```python
from build123d import *

# Parameters (mm, degrees)
SKETCH001_W           = 9.26
SKETCH001_H           = 10.18
EXTRUDE001_DEPTH      = 1.355
EXTRUDE001_DEPTH_BACK = 0.3
SKETCH002_W           = 9.26
SKETCH002_H           = 10.18
EXTRUDE002_DEPTH      = 1.35
EXTRUDE002_DEPTH_BACK = 0.3
SKETCH003_R           = 0.3
EXTRUDE003_DEPTH      = 4
EXTRUDE_DEPTH         = 59.5


with BuildPart() as extrude001:
    # Sketch001 (on Face14 of Extrude) → Extrude001 (new body, two sides)
    with BuildSketch(Plane.XY.offset(59.5)) as extrude001_sk:
        with Locations((0, 10.39)):
            Rectangle(SKETCH001_W, SKETCH001_H)
    extrude(amount=EXTRUDE001_DEPTH)
    extrude(extrude001_sk.sketch, amount=-EXTRUDE001_DEPTH_BACK)


with BuildPart() as extrude002:
    # Sketch002 (on Face13 of Extrude) → Extrude002 (new body, two sides)
    with BuildSketch(Plane(origin=(0, 0, 0), x_dir=(1, 0, 0), z_dir=(0, 0, -1))) as extrude002_sk:
        with Locations((0, -10.39)):
            Rectangle(SKETCH002_W, SKETCH002_H)
    extrude(amount=EXTRUDE002_DEPTH)
    extrude(extrude002_sk.sketch, amount=-EXTRUDE002_DEPTH_BACK)


with BuildPart() as extrude003:
    # Sketch003 (on Face4 of Extrude) → Extrude003 (new body)
    with BuildSketch(Plane.XZ):
        with Locations((-2.54, 56.42)):
            Circle(SKETCH003_R)
        with Locations((-2.54, 53.88)):
            Circle(SKETCH003_R)
        with Locations((-2.54, 51.34)):
            Circle(SKETCH003_R)
        with Locations((-2.54, 48.8)):
            Circle(SKETCH003_R)
        with Locations((-2.54, 46.26)):
            Circle(SKETCH003_R)
        with Locations((-2.54, 43.72)):
            Circle(SKETCH003_R)
        with Locations((-2.54, 41.18)):
            Circle(SKETCH003_R)
        with Locations((-2.54, 38.64)):
            Circle(SKETCH003_R)
        with Locations((-2.54, 36.1)):
            Circle(SKETCH003_R)
        with Locations((-2.54, 33.56)):
            Circle(SKETCH003_R)
        with Locations((-2.54, 31.02)):
            Circle(SKETCH003_R)
        with Locations((-2.54, 28.48)):
            Circle(SKETCH003_R)
        with Locations((-2.54, 25.94)):
            Circle(SKETCH003_R)
        with Locations((-2.54, 23.4)):
            Circle(SKETCH003_R)
        with Locations((2.54, 23.4)):
            Circle(SKETCH003_R)
        with Locations((2.54, 25.94)):
            Circle(SKETCH003_R)
        with Locations((2.54, 28.48)):
            Circle(SKETCH003_R)
        with Locations((2.54, 31.02)):
            Circle(SKETCH003_R)
        with Locations((2.54, 33.56)):
            Circle(SKETCH003_R)
        with Locations((2.54, 36.1)):
            Circle(SKETCH003_R)
        with Locations((2.54, 38.64)):
            Circle(SKETCH003_R)
        with Locations((2.54, 41.18)):
            Circle(SKETCH003_R)
        with Locations((2.54, 43.72)):
            Circle(SKETCH003_R)
        with Locations((2.54, 46.26)):
            Circle(SKETCH003_R)
        with Locations((2.54, 48.8)):
            Circle(SKETCH003_R)
        with Locations((2.54, 51.34)):
            Circle(SKETCH003_R)
        with Locations((2.54, 53.88)):
            Circle(SKETCH003_R)
        with Locations((2.54, 56.42)):
            Circle(SKETCH003_R)
        with Locations((2.54, 10.7)):
            Circle(SKETCH003_R)
        with Locations((2.54, 13.24)):
            Circle(SKETCH003_R)
        with Locations((2.54, 15.78)):
            Circle(SKETCH003_R)
        with Locations((2.54, 18.32)):
            Circle(SKETCH003_R)
        with Locations((2.54, 20.86)):
            Circle(SKETCH003_R)
        with Locations((2.54, 3.08)):
            Circle(SKETCH003_R)
        with Locations((2.54, 5.62)):
            Circle(SKETCH003_R)
        with Locations((2.54, 8.16)):
            Circle(SKETCH003_R)
        with Locations((-2.54, 10.7)):
            Circle(SKETCH003_R)
        with Locations((-2.54, 13.24)):
            Circle(SKETCH003_R)
        with Locations((-2.54, 15.78)):
            Circle(SKETCH003_R)
        with Locations((-2.54, 18.32)):
            Circle(SKETCH003_R)
        with Locations((-2.54, 20.86)):
            Circle(SKETCH003_R)
        with Locations((-2.54, 3.08)):
            Circle(SKETCH003_R)
        with Locations((-2.54, 5.62)):
            Circle(SKETCH003_R)
        with Locations((-2.54, 8.16)):
            Circle(SKETCH003_R)
    extrude(amount=EXTRUDE003_DEPTH)


with BuildPart() as fusion:
    # Sketch → Extrude (new body)
    with BuildSketch(Plane.XY):
        Polygon((-4.63, 15.48), (-4.63, 5.3), (-3.735, 5.3), (-3.735, 0), (3.735, 0), (3.735, 5.3), (4.63, 5.3), (4.63, 15.48), (1.17, 15.48), (1.17, 8.6), (-1.17, 8.6), (-1.17, 15.48), align=None)
    extrude(amount=EXTRUDE_DEPTH)

    # Fusion: union Extrude001, Extrude002, Extrude003
    add(extrude001.part)
    add(extrude002.part)
    add(extrude003.part)


solid = fusion.part
```
Source: CAD feature listing. Evaluate the final solid. Frame: model axes, mm. A direction names the side the tool comes from. Round coordinates to 2 decimals unless told otherwise and drop trailing zeros. Loops run counter-clockwise (first coordinate to the right, second up) from the corner with the lowest first, then second, coordinate; pieces in that order, holes last.
1. Section query C-C on z = 4. Output: boundary loops of the cut face in (x, y) (3 decimals), and give its area (3 significant figures).
2. Section query A-A on y = 10.5. Output: boundary loops of the cut face in (x, z) (3 decimals), and give its area (3 significant figures).
3. Mould query, pull axis X, two halves, no side actions, for faces 1 (the flat face through (0, 10, 60.855)), 2 (the flat face through (0, 12, 59.2)), 3 (the flat face through (-4.63, 10, 29)). Classes: released by +X, released by -X, zero draft, split by the parting line, or undercut.
4. Access query for faces 4 (the flat face through (0, 3, 0)), 5 (the flat face through (0, 12, 0.3)), 6 (the flat face through (0, 0, 29)), 7 (the flat face through (3.735, 3, 29)), 8 (the flat face through (0, 3, 59.5)). Directions: +Z, -Z, +X, -X, +Y, -Y. A direction counts if a zero-diameter tool reaches every point of the face in a straight line with its end or side. Return the directions, or none.
5. Section query D-D on y = -2.25. Give the number of separate pieces and of enclosed holes in the cut face, and give its area (3 significant figures).
6. Ray query, L1, parallel to X at y = 11.5, z = 41; L2, parallel to Y at x = 4, z = 36; L3, parallel to Y at x = 0.25, z = 17. Return the intervals inside material, ascending.
7. Section query B-B on x = -0.5. Output: boundary loops of the cut face in (y, z) (3 decimals).
8. Contact query for flat-ended pins moving along their axis: pin 1 (1.2 mm diameter, centred on x = 0, z = 40.5, fed in from +Y); pin 2 (4 mm diameter, centred on x = -0.5, y = 2.5, fed in from +Z); pin 3 (3 mm diameter, centred on y = -1, z = 30.5, fed in from -X) (3 decimals). Output: stop coordinate, or through.
Answers below:
1. outline: (-4.63, 5.3) - (-3.735, 5.3) - (-3.735, 0) - (3.735, 0) - (3.735, 5.3) - (4.63, 5.3) - (4.63, 15.48) - (1.17, 15.48) - (1.17, 8.6) - (-1.17, 8.6) - (-1.17, 15.48) - (-4.63, 15.48) - close
1. area: 118 mm2
2. outline: (-4.63, -1.35) - (4.63, -1.35) - (4.63, 60.855) - (-4.63, 60.855) - close; hole (-1.17, 0.3) - (1.17, 0.3) - (1.17, 59.2) - (-1.17, 59.2) - close
2. area: 438 mm2
3. face 1: zero draft
3. face 2: undercut
3. face 3: released by -X
4. face 4: -Z, +X, -X, -Y
4. face 5: +Y
4. face 6: -Y
4. face 7: +Z, -Z, +X, -Y
4. face 8: +Z, +X, -X, -Y
5. separate pieces: 44
5. enclosed holes: 0
5. area: 12.4 mm2
6. L1: x = -4.63 to -1.17, 1.17 to 4.63
6. L2: y = 5.3 to 15.48
6. L3: y = 0 to 8.6
7. outline: (0, 0) - (5.3, 0) - (5.3, -1.35) - (15.48, -1.35) - (15.48, 0.3) - (8.6, 0.3) - (8.6, 59.2) - (15.48, 59.2) - (15.48, 60.855) - (5.3, 60.855) - (5.3, 59.5) - (0, 59.5) - close
8. pin 1: stops at y = 8.6
8. pin 2: stops at z = 59.5
8. pin 3: stops at x = -3.735
